Input: part model. Units: mm. Frame: model coordinates. A direction names the side the tool comes from. Coordinates: 2 decimals unless noted, no trailing zeros. Order: outer loops, then holes, each group sorted by start corner. A loop starts at its lowest first (then second) coordinate and runs counter-clockwise, first axis right, second up. Notation, with made-up numbers: (-17, -20.75) -> (32, -20.75) arc R14 cw to (32, -12.75) -> close; hole circle Ø2 at (42, 60.5). An arc over 180 degrees is marked (long way). Use CSV: the item, a comma, the result in double quotes. Start each with the question number.
```python
from build123d import *


with BuildPart() as part:
    # Esquisse1 → Base-Révolution (revolve)
    with BuildSketch(Plane.XY, mode=Mode.PRIVATE) as base_r_volution_sk:
        with BuildLine():
            Line((0, 12), (22, 12))
            Line((22, 12), (23, 11))
            Line((23, 11), (23, 9))
            Line((23, 9), (21, 9))
            Line((21, 9), (21, 7))
            Line((21, 7), (19, 7))
            Line((19, 7), (19, 9.5))
            ThreePointArc((19, 9.5), (18.853553391, 9.853553391), (18.5, 10))
            Line((18.5, 10), (0, 10))
            Line((0, 10), (0, 12))
        make_face()
    revolve(base_r_volution_sk.sketch.rotate(Axis((0, 60, 0), (0, -1, 0)), 90), axis=Axis((0, 60, 0), (0, -1, 0)))


solid = part.part
```
1. Access query for faces 1 (the face through (11, 7, -16)), 2 (the face through (18.548, 8.268, -4.119)). Directions: +Z, -Z, +X, -X, +Y, -Y. A direction counts if a zero-diameter tool reaches every point of the face in a straight line with its end or side. Return the directions, or none.
2. Pull-direction query (X, two-part tool) for faces 3 (the face through (-22.804, 9.986, -2.994)), 4 (the face through (19, 9, 10)), 5 (the face through (0, 10, 0)); classes: released by +X, released by -X, zero draft, split by the parting line, or undercut.
3. Section A-A on x = 0. Return loops of the section in (y, z).
4. Section B-B on z = 0. Return loops of the section in (x, y), then the cut area to 3 significant figures.
5. Section C-C on y = 8. Return loops of the section in (x, z), then the cut area to 3 significant figures.
6. Material intervals for line 1 along X through (y, z) = (8.2, 0); line 2 along Y through (x, z) = (15, 9); line 3 along Y through (x, z) = (-13, 17.5), sorted ascending.
7. Contact query for flat-ended pins moving along their axis: P1, Ø1, axis at y = 11.5, z = -8, coming from the -X side; P2, Ø1.5, axis at y = 10, z = -3, coming from the -X side; P3, Ø3, axis at x = 3.5, y = 11, coming from the -Z side. Output: stop coordinate, or through.
Values follow:
1,face 1,"+Z, -Z, +X, -X, -Y"
1,face 2,"-Y"
2,face 3,"split by the parting line"
2,face 4,"zero draft"
2,face 5,"undercut"
3,outline,"(7, -21) -> (9, -21) -> (9, -23) -> (11, -23) -> (12, -22) -> (12, 22) -> (11, 23) -> (9, 23) -> (9, 21) -> (7, 21) -> (7, 19) -> (9.5, 19) arc R0.5 cw to (10, 18.5) -> (10, -18.5) arc R0.5 cw to (9.5, -19) -> (7, -19) -> close"
4,outline,"(-23, 9) -> (-21, 9) -> (-21, 7) -> (-19, 7) -> (-19, 9.5) arc R0.5 cw to (-18.5, 10) -> (18.5, 10) arc R0.5 cw to (19, 9.5) -> (19, 7) -> (21, 7) -> (21, 9) -> (23, 9) -> (23, 11) -> (22, 12) -> (-22, 12) -> (-23, 11) -> close"
4,area,"107 mm2"
5,outline,"circle Ø42 at (0, 0); hole circle Ø38 at (0, 0)"
5,area,"251 mm2"
6,line 1,"x = -21 to -19, 19 to 21"
6,line 2,"y = 10 to 12"
6,line 3,"y = 9 to 12"
7,P1,"stops at x = -21.59"
7,P2,"stops at x = -22.89"
7,P3,"stops at z = -22.91"
